Verification items for the finished model (mm, model axes). Give positions to 0.01 mm unless a question says otherwise; leave off trailing zeros. Order: outer loops, then holes, each group sorted by start corner. A loop starts at its lowest first (then second) coordinate and runs counter-clockwise, first axis right, second up.
(1) Gauge pin test, flat end, axial feed: pin 1 (5.5 mm diameter, centred on x = 6.35, y = 38.1, fed in from -Z). Record the tip position at first contact, or that the pin passes through.
(2) Sectioned sample at B-B on y = 44.45. Record the cut outline in (x, z), plus the area to 3 significant figures.
(3) Mould release check, pull along X, two halves, no side actions. Record for faces 1 (the face through (44.027, 61.767, 0.783)), 2 (the face through (65.825, 44.966, 0.783)), 3 (the face through (125.16, -30.81, 0.78)), 4 (the face through (60, 17, 1.588)): pulls with the +X half, pulls with the -X half, needs draft (parallel to the pull), parting line crosses it, or undercut.
(4) Sectioned sample at C-C on z = 0.85. Count the separate pieces of the cut face and the enclosed holes in it, plus the area to 3 significant figures.
(5) Sectioned sample at D-D on x = 130. Record the cut outline in (y, z), plus the area to 3 significant figures.
(6) Scan lines: L1, parallel to X at y = 50.8, z = 0.7; L2, parallel to X at y = 37.5, z = 1.25; L3, parallel to Y at x = 82.55, z = 0.9. Record each from-to range of solid material in increasing order.
(7) Sectioned sample at A-A on x = 63.5. Record the cut outline in (y, z).
Autodesk Inventor part; units mm, degrees
ref_plane "YZ Plane" through (0, 0, 0) normal (1, 0, 0) x (0, 1, 0)
ref_plane "XZ Plane" through (0, 0, 0) normal (0, 1, 0) x (-1, 0, 0)
ref_plane "XY Plane" through (0, 0, 0) normal (0, 0, 1) x (1, 0, 0)
sketch "Sketch1" plane through (0, 0, 0) normal (0, 0, 1) x (1, 0, 0)
  line L0 (127, 63.5) -> (127, 57.15)
  line L1 (127, 57.15) -> (127, 31.75)
  line L2 (127, 31.75) -> (152.4, 31.75)
  line L3 (0, 60.325) -> (0, 63.5)
  line L4 (0, 63.5) -> (0, 57.15)
  arc A0 (152.4, 57.15) -> (127, 31.75) centre (152.4, 31.75) ccw construction
  line L5 (127, 63.5) -> (152.4, 63.5) construction
  line L6 (152.4, 57.15) -> (152.4, 63.5) construction
  arc A1 (152.4, 57.15) -> (152.4, 63.5) centre (152.4, 60.325) ccw construction
  line L7 (127, 63.5) -> (88.9, 63.5) construction
  line L8 (0, 57.15) -> (1.3137, 57.15)
  line L9 (3.175, 57.15) -> (3.175, 53.975)
  arc A2 (3.175, 57.15) -> (0, 53.975) centre (3.175, 53.975) ccw
  arc A3 (84.3846, 63.4825) -> (4.9889, 57.4173) centre (88.9, -518.3187) ccw
  arc A4 (4.9889, 57.4173) -> (0.7473, 55.0582) centre (5.9749, 50.6519) ccw
  arc A5 (0.7473, 55.0582) -> (0, 53.0119) centre (3.175, 53.0119) ccw
  circle A6 centre (152.4, 60.325) radius 4.7625
  arc A7 (152.1428, 55.5695) -> (127, 31.75) centre (150.8543, 31.75) ccw
  line L10 (127, 60.325) -> (152.4, 60.325) construction
  arc A8 (152.4, 65.0875) -> (93.6534, 63.766) centre (144.3966, -885.5701) ccw
  arc A9 (84.3846, 63.4825) -> (93.6534, 63.766) centre (82.8076, 266.6764) ccw
  line L11 (0, 57.15) -> (0, 31.75)
  line L12 (0, 31.75) -> (0, -28.575)
  line L13 (127, 31.75) -> (126.0787, -28.6234)
  line L14 (122.9041, -31.75) -> (3.175, -31.75)
  arc A10 (0, -28.575) -> (3.175, -31.75) centre (3.175, -28.575) ccw
  arc A11 (122.9041, -31.75) -> (126.0787, -28.6234) centre (122.9041, -28.575) ccw
  point P0 (127, 44.45)
  point P1 (0, -31.75)
  point P2 (126.031, -31.75)
  point P3 (0, 53.0119)
  dimension "d15" = 6.35
  dimension "d23" = 25.4
  dimension "d24" = 25.4
  dimension "d25" = 6.35
  dimension "d27" = 0
  dimension "d28" = 38.1
  dimension "d29" = 3.175
  dimension "d31" = 3.175
  dimension "d39" = 9.525
  dimension "d40" = 203.2
  dimension "d41" = 25.4
  dimension "d42" = 63.5
  dimension "d43" = 3.175
extrude "Extrusion1" add sketch "Sketch1" along normal blind 1.5875 contours A4 A3 A9 A8 A6 A7 L13 A11 L14 A10 L12 L11 A5 | A6
sketch "Sketch2" plane through (0, 0, 1.5875) normal (0, 0, 1) x (1, 0, 0)
  line L0 (127, 63.5) -> (0, 63.5)
  line L1 (0, 63.5) -> (0, 50.8)
  line L2 (0, 63.5) -> (0, 0)
  line L3 (0, 50.8) -> (6.35, 50.8)
  line L4 (6.35, 50.8) -> (6.35, 38.1)
  line L5 (6.35, 50.8) -> (120.65, 50.8)
  line L6 (120.65, 50.8) -> (120.65, 38.1)
  line L7 (63.5, 50.8) -> (63.5, 44.45)
  line L8 (127, 63.5) -> (127, 60.325)
  line L9 (127, 60.325) -> (151.892, 60.325)
  line L10 (120.65, 38.1) -> (82.55, 38.1)
  line L11 (6.35, 38.1) -> (44.45, 38.1)
  point P0 (0, 60.325)
  point P1 (3.175, 63.5)
  dimension "d4" = 12.7
  dimension "d5" = 6.35
  dimension "d6" = 12.7
  dimension "d7" = 114.3
  dimension "d32" = 3.175
  dimension "d33" = 24.892
  dimension "d34" = 38.1
  dimension "d35" = 38.1
hole "Hole1" at (6.35, 38.1, 1.5875) at (6.35, 50.8, 1.5875) at (120.65, 38.1, 1.5875) at (120.65, 50.8, 1.5875) at (63.5, 44.45, 1.5875) at (151.892, 60.325, 1.5875) at (44.45, 38.1, 1.5875) at (82.55, 38.1, 1.5875) direction (0, 0, -1) diameter 4.7625 end through all
sketch "Sketch3" plane through (0, 0, 1.5875) normal (0, 0, 1) x (1, 0, 0)
  line L0 (0, 0) -> (0, 31.75)
  line L1 (0, 53.0119) -> (0, 3.175)
  line L2 (127, 3.175) -> (127, 31.75)
  line L3 (0, 31.75) -> (127, 31.75)
  dimension "d36" = 31.75
feature "Bend Part1" [suppressed]
properties part number "wings" material "Polycarbonate, Clear"
Ans:
1. pin 1: stops at z = 0
2. outline: (0, 0) - (61.12, 0) - (61.12, 1.59) - (0, 1.59) - close; (65.88, 0) - (130.66, 0) - (130.66, 1.59) - (65.88, 1.59) - close
2. area: 200 mm2
3. face 1: pulls with the -X half
3. face 2: undercut
3. face 3: pulls with the +X half
3. face 4: needs draft
4. separate pieces: 1
4. enclosed holes: 8
4. area: 12,100 mm2
5. outline: (43.33, 0) - (65.01, 0) - (65.01, 1.59) - (43.33, 1.59) - close
5. area: 34.4 mm2
6. L1: x = 0 to 3.97, 8.73 to 118.27, 123.03 to 136.5
6. L2: x = 0 to 4.05, 8.65 to 42.15, 46.75 to 80.25, 84.85 to 118.35, 122.95 to 127.7
6. L3: y = -31.75 to 35.72, 40.48 to 63.47
7. outline: (-31.75, 0) - (42.07, 0) - (42.07, 1.59) - (-31.75, 1.59) - close; (46.83, 0) - (62.95, 0) - (62.95, 1.59) - (46.83, 1.59) - close
